from build123d import *

# Parameters (mm, degrees)
TUBE_SQUARE_40_X_40_X_3_2_3_DEPTH = 1920
SKETCH13_R                        = 8
CUT_EXTRUDE1_DEPTH                = 1921.52076271


with BuildPart() as part:
    # Sketch12 → Tube (square) 40 X 40 X 3.2(3) (new body)
    with BuildSketch(Plane(origin=(0, 0, 0), x_dir=(0, 0, -1), z_dir=(1, 0, 0))):
        with BuildLine():
            Line((-13.6, -20), (13.6, -20))
            ThreePointArc((13.6, -20), (18.1254834, -18.1254834), (20, -13.6))
            Line((20, -13.6), (20, 13.6))
            ThreePointArc((20, 13.6), (18.1254834, 18.1254834), (13.6, 20))
            Line((13.6, 20), (-13.6, 20))
            ThreePointArc((-13.6, 20), (-18.1254834, 18.1254834), (-20, 13.6))
            Line((-20, 13.6), (-20, -13.6))
            ThreePointArc((-20, -13.6), (-18.1254834, -18.1254834), (-13.6, -20))
        make_face()
        with BuildLine():
            Line((-13.6, -16.8), (13.6, -16.8))
            ThreePointArc((13.6, -16.8), (15.8627417, -15.8627417), (16.8, -13.6))
            Line((16.8, -13.6), (16.8, 13.6))
            ThreePointArc((16.8, 13.6), (15.8627417, 15.8627417), (13.6, 16.8))
            Line((13.6, 16.8), (-13.6, 16.8))
            ThreePointArc((-13.6, 16.8), (-15.8627417, 15.8627417), (-16.8, 13.6))
            Line((-16.8, 13.6), (-16.8, -13.6))
            ThreePointArc((-16.8, -13.6), (-15.8627417, -15.8627417), (-13.6, -16.8))
        make_face(mode=Mode.SUBTRACT)
    extrude(amount=TUBE_SQUARE_40_X_40_X_3_2_3_DEPTH)

    # Sketch13 → Cut-Extrude1 (cut, through all)
    with BuildSketch(Plane(origin=(0, 20, 0), x_dir=(1, 0, 0), z_dir=(0, 1, 0))):
        with Locations(Location((220, 0, 0), (0, 0, 270))):
            Circle(SKETCH13_R)
        with Locations(Location((1700, 0, 0), (0, 0, 270))):
            Circle(SKETCH13_R)
        with Locations(Location((100, 0, 0), (0, 0, 270))):
            Circle(SKETCH13_R)
        with Locations(Location((1820, 0, 0), (0, 0, 270))):
            Circle(SKETCH13_R)
    extrude(amount=-CUT_EXTRUDE1_DEPTH, mode=Mode.SUBTRACT)


solid = part.part
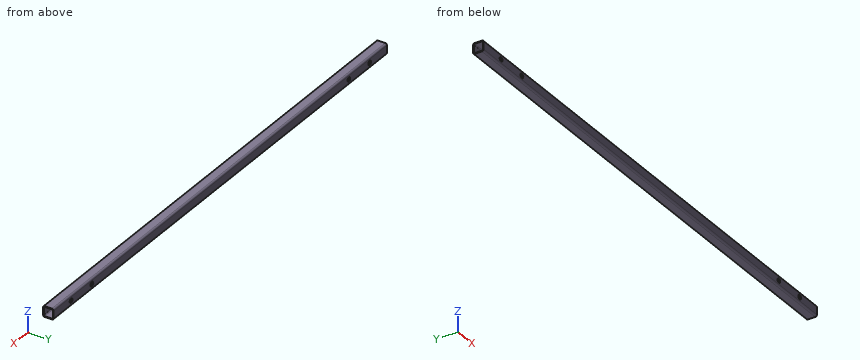
Input: part model. Units: mm. Frame: model coordinates. Give positions to 0.01 mm unless a question says otherwise; leave off trailing zeros. Loops run counter-clockwise (first coordinate to the right, second up) from the corner with the lowest first, then second, coordinate; pieces in that order, holes last. Notation, with made-up numbers: (40.5, -18) -> (89.5, -18) arc R24 ccw to (89.5, 16) -> close; hole circle Ø10 at (3, 13.5). An arc over 180 degrees is marked (long way). Answer as a JSON object with one key per item and string values. Group by question number.
Item 1: Cut plane C-C, the plane z = 0. State how many separate pieces and enclosed holes the cut face has, and give its area (3 significant figures).
Item 2: Cut plane B-B, the plane x = 913. Return the cut outline in (y, z), and give its area (3 significant figures).
Item 3: Pin query (flat end, axial travel): P1, Ø13, axis at x = 220, z = 0, coming from the +Y side. Return the tip coordinate at first contact, or that it passes through.
Item 4: Line query: probe 1 along X at (y, z) = (17.5, 0); probe 2 along Z at (x, y) = (999, -8); probe 3 along Y at (x, z) = (468, 14). Output: solid intervals per line, ascending.
Item 5: Cut plane A-A, the plane y = 7. Return the cut outline in (x, z), and give its area (3 significant figures).
Checks:
{
 "1": {"separate pieces": "10", "enclosed holes": "0", "area": "11,900 mm²"},
 "2": {"outline": "(-20, -13.6) arc R6.4 ccw to (-13.6, -20) -> (13.6, -20) arc R6.4 ccw to (20, -13.6) -> (20, 13.6) arc R6.4 ccw to (13.6, 20) -> (-13.6, 20) arc R6.4 ccw to (-20, 13.6) -> close; hole (-16.8, -13.6) arc R3.2 ccw to (-13.6, -16.8) -> (13.6, -16.8) arc R3.2 ccw to (16.8, -13.6) -> (16.8, 13.6) arc R3.2 ccw to (13.6, 16.8) -> (-13.6, 16.8) arc R3.2 ccw to (-16.8, 13.6) -> close", "area": "445 mm²"},
 "3": {"P1": "passes through"},
 "4": {"probe 1": "x = 0 to 92, 108 to 212, 228 to 1692, 1708 to 1812, 1828 to 1920", "probe 2": "z = -20 to -16.8, 16.8 to 20", "probe 3": "y = -19.99 to -16.77, 16.77 to 19.99"},
 "5": {"outline": "(0, -20) -> (1920, -20) -> (1920, -16.8) -> (0, -16.8) -> close; (0, 16.8) -> (1920, 16.8) -> (1920, 20) -> (0, 20) -> close", "area": "12,300 mm²"}
}
